from build123d import *

# Parameters (mm, degrees)
SKETCH2_R             = 4.5
SKETCH2_R_2           = 1.5
BOSS_EXTRUDE1_DEPTH   = 10
BOSS_EXTRUDE1_2_DEPTH = 10
BOSS_EXTRUDE1_3_DEPTH = 10
BOSS_EXTRUDE1_4_DEPTH = 10
SKETCH3_W             = 85
SKETCH3_H             = 65
BOSS_EXTRUDE2_DEPTH   = 3


with BuildPart() as part:
    # Sketch2 → Boss-Extrude1 (new body)
    with BuildSketch(Plane(origin=(0, 0, 0), x_dir=(1, 0, 0), z_dir=(0, 1, 0))):
        with Locations(Location((66, 8, 0), (0, 0, 270))):
            Circle(SKETCH2_R)
        with Locations(Location((66, 8, 0), (0, 0, 270))):
            Circle(SKETCH2_R_2, mode=Mode.SUBTRACT)
    extrude(amount=BOSS_EXTRUDE1_DEPTH)



with BuildPart() as body_2:
    # Sketch2 → Boss-Extrude1 2 (new body)
    with BuildSketch(Plane(origin=(0, 0, 0), x_dir=(1, 0, 0), z_dir=(0, 1, 0))):
        with Locations(Location((66, 57, 0), (0, 0, 270))):
            Circle(SKETCH2_R)
        with Locations(Location((66, 57, 0), (0, 0, 270))):
            Circle(SKETCH2_R_2, mode=Mode.SUBTRACT)
    extrude(amount=BOSS_EXTRUDE1_2_DEPTH)


with BuildPart() as body_3:
    # Sketch2 → Boss-Extrude1 3 (new body)
    with BuildSketch(Plane(origin=(0, 0, 0), x_dir=(1, 0, 0), z_dir=(0, 1, 0))):
        with Locations(Location((8, 57, 0), (0, 0, 270))):
            Circle(SKETCH2_R)
        with Locations(Location((8, 57, 0), (0, 0, 270))):
            Circle(SKETCH2_R_2, mode=Mode.SUBTRACT)
    extrude(amount=BOSS_EXTRUDE1_3_DEPTH)


with BuildPart() as body_4:
    # Sketch2 → Boss-Extrude1 4 (new body)
    with BuildSketch(Plane(origin=(0, 0, 0), x_dir=(1, 0, 0), z_dir=(0, 1, 0))):
        with Locations(Location((8, 8, 0), (0, 0, 270))):
            Circle(SKETCH2_R)
        with Locations(Location((8, 8, 0), (0, 0, 270))):
            Circle(SKETCH2_R_2, mode=Mode.SUBTRACT)
    extrude(amount=BOSS_EXTRUDE1_4_DEPTH)


with BuildPart() as part_1:
    add(part.part)

    add(body_2.part)  # Boss-Extrude2 merges body 2

    add(body_3.part)  # Boss-Extrude2 merges body 3

    add(body_4.part)  # Boss-Extrude2 merges body 4
    # Sketch3 → Boss-Extrude2 (add)
    with BuildSketch(Plane(origin=(0, 0, 0), x_dir=(1, 0, 0), z_dir=(0, 1, 0))):
        with Locations((42.5, 32.5)):
            Rectangle(SKETCH3_W, SKETCH3_H)
    extrude(amount=-BOSS_EXTRUDE2_DEPTH)


solid = part_1.part
Check sheet for the modelled part. Datum: model origin and axes. Units: mm. A direction names the side the tool comes from. Give positions to 0.01 mm unless a question says otherwise; leave off trailing zeros. Write each loop counter-clockwise with the first axis right and the second up, starting at its lowest first coordinate (ties: lowest second). Pieces come first, ordered by that corner, then holes. Notation, with made-up numbers: (78.5, 86) -> (135.5, 86) arc R24 cw to (135.5, 118) -> close; hole circle Ø9 at (-5, 48). An arc over 180 degrees is marked (long way). Use one line per item in the form item = value. Start each with the question number.
1. Access from +Z, -Z, +X, -X, +Y, -Y to the whole of each face (thin tool, end or side, straight path). Record for faces 4 (the cylindrical face through (9.352, 4.93, -3.708)), 5 (the flat face through (42, -1, -65)).
2. Section check D-D (x = 22.5). Record the cut outline in (y, z).
3. Section check C-C (z = -8). Record the cut outline in (x, y), and give its area (3 significant figures).
4. Go/stop test with a flat-tipped pin: P1, Ø4, axis at x = 38, z = -35, coming from the +Y side. Record where the tip stops, or that it passes through.
5. Mould release check, pull along Z, two halves, no side actions. Record for faces 1 (the flat face through (8, 0, -57)), 2 (the flat face through (42, -1, 0)), 3 (the flat face through (66, 10, -6)): pulls with the +Z half, pulls with the -Z half, needs draft (parallel to the pull), parting line crosses it, or undercut.
6. Section check B-B (x = 66). Record the cut outline in (y, z), and give its area (3 significant figures).
7. Thickness scan on line 1 along X through (y, z) = (3, -8); line 2 along X through (y, z) = (4.5, -56); line 3 along Y through (x, z) = (66, -26). Record the ranges inside material, lowest first. Write a range as from..to.
8. Section check A-A (y = 8.5). Record the cut outline in (x, z).
Conclusion:
q1.face_4 = +Y
q1.face_5 = -Z, +X, -X, +Y, -Y
q2.outline = (-3, -65) -> (0, -65) -> (0, 0) -> (-3, 0) -> close
q3.outline = (0, -3) -> (85, -3) -> (85, 0) -> (70.5, 0) -> (70.5, 10) -> (67.5, 10) -> (67.5, 0) -> (64.5, 0) -> (64.5, 10) -> (61.5, 10) -> (61.5, 0) -> (12.5, 0) -> (12.5, 10) -> (9.5, 10) -> (9.5, 0) -> (6.5, 0) -> (6.5, 10) -> (3.5, 10) -> (3.5, 0) -> (0, 0) -> close
q3.area = 375 mm²
q4.P1 = 0
q5.face_1 = undercut
q5.face_2 = pulls with the +Z half
q5.face_3 = needs draft
q6.outline = (-3, -65) -> (0, -65) -> (0, -61.5) -> (10, -61.5) -> (10, -58.5) -> (0, -58.5) -> (0, -55.5) -> (10, -55.5) -> (10, -52.5) -> (0, -52.5) -> (0, -12.5) -> (10, -12.5) -> (10, -9.5) -> (0, -9.5) -> (0, -6.5) -> (10, -6.5) -> (10, -3.5) -> (0, -3.5) -> (0, 0) -> (-3, 0) -> close
q6.area = 315 mm²
q7.line_1 = 3.5..6.5, 9.5..12.5, 61.5..64.5, 67.5..70.5
q7.line_2 = 3.61..6.88, 9.12..12.39, 61.61..64.88, 67.12..70.39
q7.line_3 = -3..0
q8.outline = circle Ø9 at (8, -57); circle Ø9 at (8, -8); circle Ø9 at (66, -57); circle Ø9 at (66, -8); hole circle Ø3 at (8, -57); hole circle Ø3 at (8, -8); hole circle Ø3 at (66, -57); hole circle Ø3 at (66, -8)
